Source: CAD feature listing. Evaluate the final solid. Frame: model axes, mm. Coordinates: 2 decimals unless noted, no trailing zeros. Loops run counter-clockwise (first coordinate to the right, second up) from the corner with the lowest first, then second, coordinate; pieces in that order, holes last. Notation, with made-up numbers: (76, 1.5) - (88, 1.5) arc R37 cw to (88, 40.5) - close; hole circle Ø2 at (79.25, -7.5). An arc over 180 degrees is marked (long way). Use CSV: the item, a comma, the result in double quotes. Start each with the question number.
```python
from build123d import *

# Parameters (mm, degrees)
F0_W     = 80
F0_H     = 80
F1_DEPTH = 5
F3_D     = 4.4
F4_R     = 10


with BuildPart() as f1:
    # F0 (on Top) → F1 (new body)
    with BuildSketch(Plane.XY):
        Rectangle(F0_W, F0_H)
    extrude(amount=F1_DEPTH)

    # F3 (through all)
    with Locations(Plane.XY.offset(5)):
        with Locations((0, 25), (21.650635, 12.5), (21.650635, -12.5), (0, -25), (-21.650635, -12.5), (-21.650635, 12.5)):
            Hole(F3_D / 2)

    # F4
    f4_edges = [f1.edges().sort_by_distance(p)[0] for p in [
        (40, -40, 2.5),
        (40, 40, 2.5),
        (-40, -40, 2.5),
        (-40, 40, 2.5),
    ]]
    fillet(f4_edges, radius=F4_R)


solid = f1.part
```
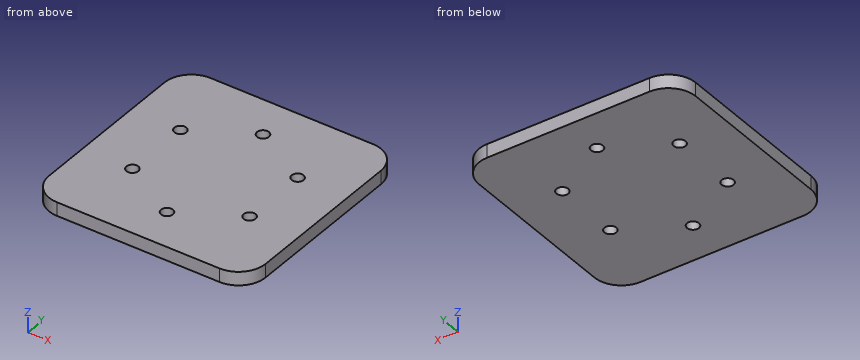
(1) Section B-B on x = 0. Output: boundary loops of the cut face in (y, z), plus the area to 3 significant figures.
(2) Ray query, line 1 (Y direction, x = 0, z = 1.25); line 2 (Y direction, x = 34, z = 1.7); line 3 (Y direction, x = 35.5, z = 3.3). Return the intervals inside material, ascending. Write a range as [from, to].
(3) Section D-D on y = 25. Output: boundary loops of the cut face in (x, z), plus the area to 3 significant figures.
(4) Section C-C on y = -12.5. Output: boundary loops of the cut face in (x, z), plus the area to 3 significant figures.
(5) Section A-A on z = 4.1. Output: boundary loops of the cut face in (x, y), plus the area to 3 significant figures.
Solution:
1,outline,"(-40, 0) - (-27.2, 0) - (-27.2, 5) - (-40, 5) - close; (-22.8, 0) - (22.8, 0) - (22.8, 5) - (-22.8, 5) - close; (27.2, 0) - (40, 0) - (40, 5) - (27.2, 5) - close"
1,area,"356 mm²"
2,line 1,"y = [-40, -27.2], [-22.8, 22.8], [27.2, 40]"
2,line 2,"y = [-39.17, 39.17]"
2,line 3,"y = [-38.35, 38.35]"
3,outline,"(-40, 0) - (-2.2, 0) - (-2.2, 5) - (-40, 5) - close; (2.2, 0) - (40, 0) - (40, 5) - (2.2, 5) - close"
3,area,"378 mm²"
4,outline,"(-40, 0) - (-23.85, 0) - (-23.85, 5) - (-40, 5) - close; (-19.45, 0) - (19.45, 0) - (19.45, 5) - (-19.45, 5) - close; (23.85, 0) - (40, 0) - (40, 5) - (23.85, 5) - close"
4,area,"356 mm²"
5,outline,"(-40, -30) arc R10 ccw to (-30, -40) - (30, -40) arc R10 ccw to (40, -30) - (40, 30) arc R10 ccw to (30, 40) - (-30, 40) arc R10 ccw to (-40, 30) - close; hole circle Ø4.4 at (-21.65, -12.5); hole circle Ø4.4 at (-21.65, 12.5); hole circle Ø4.4 at (0, -25); hole circle Ø4.4 at (0, 25); hole circle Ø4.4 at (21.65, -12.5); hole circle Ø4.4 at (21.65, 12.5)"
5,area,"6,220 mm²"
